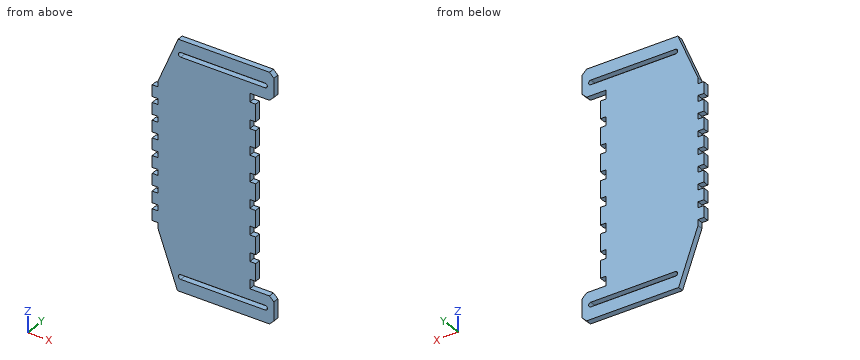
Autodesk Inventor part; units mm, degrees
ref_plane "YZ Plane" through (0, 0, 0) normal (1, 0, 0) x (0, 1, 0)
ref_plane "XZ Plane" through (0, 0, 0) normal (0, 1, 0) x (-1, 0, 0)
ref_plane "XY Plane" through (0, 0, 0) normal (0, 0, 1) x (1, 0, 0)
sketch "Эскиз1" plane through (0, 0, 0) normal (0, 1, 0) x (-1, 0, 0)
  line L0 (-37.5, 85.25) -> (37.5, 85.25)
  line L1 (37.5, 85.25) -> (37.5, -85.25)
  line L2 (37.5, -85.25) -> (-37.5, -85.25)
  line L3 (-37.5, -85.25) -> (-37.5, 85.25)
  line L4 (-37.5, 85.25) -> (37.5, -85.25) construction
  line L5 (37.5, 85.25) -> (-37.5, -85.25) construction
  circle A0 centre (21.5, 75.25) radius 1.6 construction
  circle A1 centre (-26.5, 75.25) radius 1.6 construction
  line L6 (37.5, 0) -> (0, 0) construction
  line L7 (-37.5, -85.25) -> (37.5, 85.25) construction
  circle A2 centre (21.5, -75.25) radius 1.6 construction
  circle A3 centre (-26.5, -75.25) radius 1.6 construction
  line L8 (37.5, 75.25) -> (-37.5, 75.25) construction
  line L9 (28.1, 75.25) -> (-33.1, 75.25) construction
  line L10 (26.5, 76.85) -> (-31.5, 76.85)
  line L11 (-31.5, 73.65) -> (26.5, 73.65)
  arc A4 (26.5, 73.65) -> (26.5, 76.85) centre (26.5, 75.25) ccw
  arc A5 (-31.5, 76.85) -> (-31.5, 73.65) centre (-31.5, 75.25) ccw
  line L12 (26.5, -76.85) -> (-31.5, -76.85)
  line L13 (-31.5, -73.65) -> (26.5, -73.65)
  arc A6 (26.5, -76.85) -> (26.5, -73.65) centre (26.5, -75.25) ccw
  arc A7 (-31.5, -73.65) -> (-31.5, -76.85) centre (-31.5, -75.25) ccw
  point P0 (-2.5, 75.25)
  point P1 (-33.1, -75.25)
  dimension "d0" = 170.5
  dimension "d1" = 75
  dimension "d2" = 3.2
  dimension "d4" = 10
  dimension "d5" = 3.2
  dimension "d7" = 10
  dimension "d29" = 48
  dimension "d30" = 3.2
  dimension "d32" = 5
  dimension "d33" = 5
  dimension "d59" = 6
  dimension "d60" = 10
extrude "Выдавливание1" add sketch "Эскиз1" along normal blind 4
sketch "Эскиз2" plane through (0, 4, 0) normal (0, 1, 0) x (1, 0, 0)
  line L0 (33, 66.25) -> (33, -66.25) construction
  line L1 (-37.5, -85.25) -> (37.5, -85.25)
  line L2 (37.5, 85.25) -> (-37.5, 85.25)
  line L3 (21, -66.25) -> (25, -66.25)
  line L4 (25, -66.25) -> (25, -60.25)
  line L5 (25, -60.25) -> (21, -60.25)
  line L6 (21, -60.25) -> (21, -66.25)
  line L7 (21, -48.25) -> (25, -48.25)
  line L8 (21, -42.25) -> (21, -48.25)
  line L9 (25, -48.25) -> (25, -42.25)
  line L10 (25, -42.25) -> (21, -42.25)
  line L11 (21, -30.25) -> (25, -30.25)
  line L12 (21, -24.25) -> (21, -30.25)
  line L13 (25, -30.25) -> (25, -24.25)
  line L14 (25, -24.25) -> (21, -24.25)
  line L15 (21, -12.25) -> (25, -12.25)
  line L16 (21, -6.25) -> (21, -12.25)
  line L17 (25, -12.25) -> (25, -6.25)
  line L18 (25, -6.25) -> (21, -6.25)
  line L19 (21, 5.75) -> (25, 5.75)
  line L20 (21, 11.75) -> (21, 5.75)
  line L21 (25, 5.75) -> (25, 11.75)
  line L22 (25, 11.75) -> (21, 11.75)
  line L23 (21, 23.75) -> (25, 23.75)
  line L24 (21, 29.75) -> (21, 23.75)
  line L25 (25, 23.75) -> (25, 29.75)
  line L26 (25, 29.75) -> (21, 29.75)
  line L27 (21, 41.75) -> (25, 41.75)
  line L28 (21, 47.75) -> (21, 41.75)
  line L29 (25, 41.75) -> (25, 47.75)
  line L30 (25, 47.75) -> (21, 47.75)
  line L31 (21, 59.75) -> (25, 59.75)
  line L32 (25, 59.75) -> (25, 66.25)
  line L33 (25, 66.25) -> (21, 66.25)
  line L34 (21, 66.25) -> (21, 59.75)
  point P0 (27, -66.25)
  dimension "d14" = 19
  dimension "d16" = 4
  dimension "d17" = 6
  dimension "d20" = 18
  dimension "d34" = 4
  dimension "d35" = 6.5
  dimension "d36" = 12
extrude "Выдавливание2" cut sketch "Эскиз2" against normal blind 10
sketch "Эскиз3" plane through (0, 4, 0) normal (0, 1, 0) x (1, 0, 0)
  line L0 (37.5, -85.25) -> (37.5, 85.25)
  line L1 (37.5, 66.25) -> (25, 66.25)
  line L2 (25, 66.25) -> (25, -66.25)
  line L3 (25, -66.25) -> (37.5, -66.25)
  line L4 (37.5, -66.25) -> (37.5, 66.25)
  line L5 (-26.5, -73.65) -> (31.5, -73.65)
  line L6 (31.5, 73.65) -> (-26.5, 73.65)
  line L7 (25, -24.25) -> (25, -30.25)
  point P0 (0, 0)
  point P1 (31.25, 66.25)
  point P2 (25, -27.25)
  point P3 (37.5, -66.25)
  point P4 (25, -66.25)
  point P5 (25, 66.25)
  dimension "d39" = 0
extrude "Выдавливание3" cut sketch "Эскиз3" against normal blind 10
chamfer "Фаска1" distance 3 angle 45 4 edges at (37.5, 2, 66.25) (37.5, 2, -66.25) (37.5, 2, -85.25) (37.5, 2, 85.25)
sketch "Эскиз5" plane through (0, 4, 0) normal (0, 1, 0) x (1, 0, 0)
  line L0 (-37.5, 85.25) -> (-37.5, -85.25)
  line L1 (-37.5, -85.25) -> (-46.1, -85.25)
  line L2 (-46.1, -85.25) -> (-46.1, 85.25)
  line L3 (-46.1, 85.25) -> (-37.5, 85.25)
  line L4 (-37.5, 85.25) -> (-37.5, -85.25)
  point P0 (0, 0)
  dimension "d61" = 8.6
extrude "Выдавливание5" add sketch "Эскиз5" against normal blind 4
sketch "Эскиз6" plane through (0, 4, 0) normal (0, 1, 0) x (1, 0, 0)
  line L0 (-46.1, -60) -> (-42.1, -60) construction
  line L1 (-42.1, 60) -> (-46.1, 60) construction
  line L2 (-46.1, 60) -> (-46.1, -60) construction
  line L3 (-46.1, -60) -> (-42.1, 60) construction
  line L4 (-42.1, -60) -> (-46.1, 60) construction
  line L5 (-46.1, 85.25) -> (-46.1, -85.25) construction
  line L6 (-42.1, -48) -> (-46.1, -48)
  line L7 (-46.1, -48) -> (-46.1, -52)
  line L8 (-46.1, -52) -> (-42.1, -52)
  line L9 (-42.1, -52) -> (-42.1, -48)
  line L10 (-42.1, -40) -> (-42.1, -36)
  line L11 (-46.1, -40) -> (-42.1, -40)
  line L12 (-46.1, -36) -> (-46.1, -40)
  line L13 (-42.1, -36) -> (-46.1, -36)
  line L14 (-42.1, -28) -> (-42.1, -24)
  line L15 (-46.1, -28) -> (-42.1, -28)
  line L16 (-46.1, -24) -> (-46.1, -28)
  line L17 (-42.1, -24) -> (-46.1, -24)
  line L18 (-42.1, -16) -> (-42.1, -12)
  line L19 (-46.1, -16) -> (-42.1, -16)
  line L20 (-46.1, -12) -> (-46.1, -16)
  line L21 (-42.1, -12) -> (-46.1, -12)
  line L22 (-42.1, -4) -> (-42.1, 0)
  line L23 (-46.1, -4) -> (-42.1, -4)
  line L24 (-46.1, 0) -> (-46.1, -4)
  line L25 (-42.1, 0) -> (-46.1, 0)
  line L26 (-42.1, 8) -> (-42.1, 12)
  line L27 (-46.1, 8) -> (-42.1, 8)
  line L28 (-46.1, 12) -> (-46.1, 8)
  line L29 (-42.1, 12) -> (-46.1, 12)
  line L30 (-42.1, 20) -> (-42.1, 24)
  line L31 (-46.1, 20) -> (-42.1, 20)
  line L32 (-46.1, 24) -> (-46.1, 20)
  line L33 (-42.1, 24) -> (-46.1, 24)
  line L34 (-42.1, 32) -> (-42.1, 36)
  line L35 (-46.1, 32) -> (-42.1, 32)
  line L36 (-46.1, 36) -> (-46.1, 32)
  line L37 (-42.1, 36) -> (-46.1, 36)
  line L38 (-42.1, 44) -> (-42.1, 48)
  line L39 (-46.1, 44) -> (-42.1, 44)
  line L40 (-46.1, 48) -> (-46.1, 44)
  line L41 (-42.1, 48) -> (-46.1, 48)
  point P0 (0, 0)
  point P1 (-44.1, 0)
  point P2 (-46.1, 0)
  dimension "d64" = 4
  dimension "d65" = 120
  dimension "d66" = 4
  dimension "d67" = 4
  dimension "d68" = 8
  dimension "d71" = 12
extrude "Выдавливание6" cut sketch "Эскиз6" against normal blind 4
sketch "Эскиз7" plane through (0, 4, 0) normal (0, 1, 0) x (1, 0, 0)
  line L0 (-42.1, -52) -> (-42.1, -48)
  line L1 (-42.1, -52) -> (-28.2738, -85.25)
  line L2 (34.5, -85.25) -> (-46.1, -85.25)
  line L3 (-46.1, -52) -> (-46.1, -85.25)
  line L4 (-46.1, -85.25) -> (-28.2738, -85.25)
  line L5 (-46.1, -85.25) -> (-46.1, -52)
  line L6 (-46.1, -52) -> (-42.1, -52)
  arc A0 (-26.5, -73.65) -> (-26.5, -76.85) centre (-26.5, -75.25) ccw
  line L7 (0, 0) -> (-4.0175, 0)
  line L8 (-42.1, 48) -> (-42.1, 44)
  line L9 (-42.1, 48) -> (-28.7698, 85.25)
  line L10 (34.5, 85.25) -> (-46.1, 85.25)
  line L11 (-46.1, 85.25) -> (-28.7698, 85.25)
  line L12 (-46.1, 85.25) -> (-46.1, 48)
  line L13 (-46.1, 48) -> (-42.1, 48)
  arc A1 (-26.5, 76.85) -> (-26.5, 73.65) centre (-26.5, 75.25) ccw
  point P0 (-28.1, -75.25)
  point P1 (-28.1, 75.25)
  dimension "d78" = 4
  dimension "d81" = 4
extrude "Выдавливание7" cut sketch "Эскиз7" against normal blind 4
properties part number "ребро_электроника"
Check sheet for the modelled part. Datum: model origin and axes. Units: mm. Round coordinates to 2 decimals unless told otherwise and drop trailing zeros. Order: outer loops, then holes, each group sorted by start corner. A loop starts at its lowest first (then second) coordinate and runs counter-clockwise, first axis right, second up.
(1) Go/stop test with flat-tipped pins: P1, Ø1.5, axis at x = -28.5, y = 2.5, coming from the +Z side; P2, Ø2, axis at y = 1.5, z = -33.5, coming from the -X side; P3, Ø1.2, axis at x = -44.5, y = 2, coming from the +Z side; P4, Ø1.2, axis at y = 2.5, z = 9, coming from the +X side. Record where each tip stops, or that it passes through.
(2) Scan lines: probe 1 along Z at (x, y) = (18.5, 2.75); probe 2 along Z at (x, y) = (26, 3.5); probe 3 along Z at (x, y) = (33.5, 3.4). Record each from-to range of solid material in increasing order.
(3) Cross-section at A-A, the plane x = 6. Enter the section's corners in (y, z).
(4) Cross-section at B-B, the plane z = 75.25. Enter the section's corners in (x, y), and give its area (3 significant figures).
(5) Cross-section at C-C, the plane y = 2. State how many separate pieces and enclosed holes the cut face has, and give its area (3 significant figures).
(6) Cross-section at D-D, the plane z = -75.25. Enter the section's corners in (x, y), and give its area (3 significant figures).
Check sheet entries:
1. P1: stops at z = 85.25
1. P2: stops at x = -42.1
1. P3: stops at z = 48
1. P4: stops at x = 21
2. probe 1: z = -85.25 to -76.85, -73.65 to 73.65, 76.85 to 85.25
2. probe 2: z = -85.25 to -76.85, -73.65 to -66.25, 66.25 to 73.65, 76.85 to 85.25
2. probe 3: z = -85.25 to -66.25, 66.25 to 85.25
3. outline: (0, -85.25) - (4, -85.25) - (4, -76.85) - (0, -76.85) - close; (0, -73.65) - (4, -73.65) - (4, 73.65) - (0, 73.65) - close; (0, 76.85) - (4, 76.85) - (4, 85.25) - (0, 85.25) - close
4. outline: (-32.43, 0) - (-28.1, 0) - (-28.1, 4) - (-32.43, 4) - close; (33.1, 0) - (37.5, 0) - (37.5, 4) - (33.1, 4) - close
4. area: 34.9 mm2
5. separate pieces: 1
5. enclosed holes: 2
5. area: 11,100 mm2
6. outline: (-32.35, 0) - (-28.1, 0) - (-28.1, 4) - (-32.35, 4) - close; (33.1, 0) - (37.5, 0) - (37.5, 4) - (33.1, 4) - close
6. area: 34.6 mm2
